Could you check a few things on this model? Use its own coordinates, in mm. A direction names the side the tool comes from. Round coordinates to 2 decimals unless told otherwise and drop trailing zeros. Write each loop counter-clockwise with the first axis right and the second up, starting at its lowest first coordinate (ties: lowest second). Pieces come first, ordered by that corner, then holes. Notation, with made-up numbers: (64.25, 46.5) - (73.25, 46.5) arc R23 ccw to (73.25, 83.5) - close; hole circle Ø4 at (36.25, -14.75). An arc over 180 degrees is marked (long way). Write each question's results on one line, items separated by ' | '. Start each with the question number.
(1) Please list where these lines run through material, in increasing order: line 1 (X direction, y = 166, z = -13.5); line 2 (Y direction, x = 503.5, z = -26.5); line 3 (Y direction, x = 641, z = -84). Write a range as [from, to].
(2) Imagine slicing it at A-A on z = -80. Write out the boundary of the cut face in (x, y).
(3) Imagine slicing it at C-C on y = 275. Write out the boundary of the cut face in (x, z).
(4) Imagine slicing it at B-B on x = 992. Write out the boundary of the cut face in (y, z).
(5) Imagine slicing it at D-D on x = 793.75. Write out the boundary of the cut face in (y, z).
(6) On a 3-axis mill with a long thin cutter (end or side, diameter ignored), from which of +Z, -Z, +X, -X, +Y, -Y can I reach the whole of each face in a straight line? I mean faces 4 (the flat face through (793, 379, -50.8)), 5 (the flat face through (617, 127, -50)), 6 (the flat face through (1042, 190.5, -19)), 7 (the flat face through (584.2, 165, -19)). Say none if no direction works.
(7) Thinking about a two-plate mould opening in X: for faces 1 (the flat face through (965.2, 165, -19)), 2 (the flat face through (914.4, 165, -19)), 3 (the flat face through (179, 190.5, -19)), which applies, +X half, -X half, draft (parallel to the pull), parting line (faces both ways), or undercut?
(8) For P1, Ø14, axis at y = 134.5, z = -34, coming from the -X side; P2, Ø8, axis at y = 142, z = -24.5, coming from the +X side; P3, Ø1.5, axis at x = 735, z = -22, coming from the +Y side, each with a flat end and sliding along its axis, tell me the tip position at first contact or that it passes through.
```python
from build123d import *

# Parameters (mm, degrees)
F0_W      = 1219.2
F0_H      = 393.7
F1_DEPTH  = 6.35
F3_DEPTH  = 6.351
F4_W      = 152.4
F4_H      = 12.7
F5_DEPTH  = 101.6
F8_DEPTH  = 50.8
F10_DEPTH = 38.1
F11_DEPTH = 101.6
F9_W      = 50.8
F9_H      = 50.8
F12_DEPTH = 38.1


with BuildPart() as f1:
    # F0 (on Top) → F1 (new body)
    with BuildSketch(Plane.XY):
        with Locations((609.6, 196.85)):
            Rectangle(F0_W, F0_H)
    extrude(amount=F1_DEPTH)

    # F2 (on face) → F3 (cut, through all)
    with BuildSketch(Plane.XY.offset(6.35)):
        with BuildLine():
            ThreePointArc((533.4, 330.2), (546.8703841816, 335.7796158184), (552.45, 349.25))
            ThreePointArc((552.45, 349.25), (546.8703841816, 362.7203841816), (533.4, 368.3))
            ThreePointArc((533.4, 368.3), (514.35, 349.25), (533.4, 330.2))
        make_face()
        with BuildLine():
            ThreePointArc((533.4, 368.3), (546.8703841816, 362.7203841816), (552.45, 349.25))
            Line((552.45, 349.25), (666.75, 349.25))
            ThreePointArc((666.75, 349.25), (672.3296158184, 362.7203841816), (685.8, 368.3))
            Line((685.8, 368.3), (533.4, 368.3))
        make_face()
        with BuildLine():
            Line((666.75, 349.25), (552.45, 349.25))
            ThreePointArc((552.45, 349.25), (546.8703841816, 335.7796158184), (533.4, 330.2))
            Line((533.4, 330.2), (685.8, 330.2))
            ThreePointArc((685.8, 330.2), (672.3296158184, 335.7796158184), (666.75, 349.25))
        make_face()
        with BuildLine():
            ThreePointArc((685.8, 368.3), (672.3296158184, 362.7203841816), (666.75, 349.25))
            ThreePointArc((666.75, 349.25), (672.3296158184, 335.7796158184), (685.8, 330.2))
            ThreePointArc((685.8, 330.2), (699.2703841816, 335.7796158184), (704.85, 349.25))
            ThreePointArc((704.85, 349.25), (699.2703841816, 362.7203841816), (685.8, 368.3))
        make_face()
    extrude(amount=-F3_DEPTH, mode=Mode.SUBTRACT)

    # F4 (on face) → F5 (join)
    with BuildSketch(Plane(origin=(0, 0, 0), x_dir=(1, 0, 0), z_dir=(0, 0, -1))):
        with Locations((609.6, -247.65)):
            Rectangle(F4_W, F4_H)
    extrude(amount=F5_DEPTH)

    # F7 (on face) → F8 (join)
    with BuildSketch(Plane(origin=(0, 0, 0), x_dir=(1, 0, 0), z_dir=(0, 0, -1))):
        with BuildLine():
            Line((133.35, -393.7), (209.55, -393.7))
            ThreePointArc((209.55, -393.7), (171.45, -355.6), (133.35, -393.7))
        make_face()
        with BuildLine():
            Line((387.35, -393.7), (463.55, -393.7))
            ThreePointArc((463.55, -393.7), (425.45, -355.6), (387.35, -393.7))
        make_face()
        with BuildLine():
            ThreePointArc((831.85, -393.7), (793.75, -355.6), (755.65, -393.7))
            Line((755.65, -393.7), (831.85, -393.7))
        make_face()
        with BuildLine():
            ThreePointArc((1085.85, -393.7), (1047.75, -355.6), (1009.65, -393.7))
            Line((1009.65, -393.7), (1085.85, -393.7))
        make_face()
    extrude(amount=F8_DEPTH)

    # F9 (on face) → F10 (join)
    with BuildSketch(Plane(origin=(0, 0, 0), x_dir=(1, 0, 0), z_dir=(0, 0, -1))):
        Polygon((304.8, -190.5), (254, -190.5), (101.6, -190.5), (101.6, -203.2), (1117.6, -203.2), (1117.6, -190.5), (965.2, -190.5), (914.4, -190.5), (635, -190.5), (584.2, -190.5), align=None)
    extrude(amount=F10_DEPTH)

    # F9 (on face) → F11 (join)
    with BuildSketch(Plane(origin=(0, 0, 0), x_dir=(1, 0, 0), z_dir=(0, 0, -1))):
        Polygon((101.6, -139.7), (254, -139.7), (304.8, -139.7), (584.2, -139.7), (635, -139.7), (914.4, -139.7), (965.2, -139.7), (1117.6, -139.7), (1117.6, -127), (101.6, -127), align=None)
    extrude(amount=F11_DEPTH)

    # F9 (on face) → F12 (join, through all)
    with BuildSketch(Plane(origin=(0, 0, 0), x_dir=(1, 0, 0), z_dir=(0, 0, -1))):
        with Locations((279.4, -165.1)):
            Rectangle(F9_W, F9_H)
        with Locations((609.6, -165.1)):
            Rectangle(F9_W, F9_H)
        with Locations((939.8, -165.1)):
            Rectangle(F9_W, F9_H)
    extrude(amount=F12_DEPTH)


solid = f1.part
```
Response:
1) line 1: [254, 304.8], [584.2, 635], [914.4, 965.2] | line 2: [127, 139.7], [190.5, 203.2] | line 3: [127, 139.7], [241.3, 254]
2) outline: (101.6, 127) - (1117.6, 127) - (1117.6, 139.7) - (101.6, 139.7) - close; (533.4, 241.3) - (685.8, 241.3) - (685.8, 254) - (533.4, 254) - close
3) outline: (0, 0) - (1219.2, 0) - (1219.2, 6.35) - (0, 6.35) - close
4) outline: (0, 0) - (127, 0) - (127, -101.6) - (139.7, -101.6) - (139.7, 0) - (190.5, 0) - (190.5, -38.1) - (203.2, -38.1) - (203.2, 0) - (393.7, 0) - (393.7, 6.35) - (0, 6.35) - close
5) outline: (0, 0) - (127, 0) - (127, -101.6) - (139.7, -101.6) - (139.7, 0) - (190.5, 0) - (190.5, -38.1) - (203.2, -38.1) - (203.2, 0) - (355.6, 0) - (355.6, -50.8) - (393.7, -50.8) - (393.7, 6.35) - (0, 6.35) - close
6) face 4: -Z, +X, -X, +Y | face 5: -Z, +X, -X, -Y | face 6: -Z, +X | face 7: -Z
7) face 1: +X half | face 2: undercut | face 3: draft
8) P1: x = 101.6 | P2: x = 1117.6 | P3: y = 203.2
